Can you work these out from the model? Positions are in its coordinate system, mm. Face numbers are marked on the shaded views. A direction names the side the tool comes from. Give positions to 0.01 mm unless a question says otherwise; leave off trailing zeros. Loops run counter-clockwise (first coordinate to the right, second up) from the corner with the lowest first, then second, coordinate; pieces in that order, holes last. Notation, with made-up numbers: (36.25, 38.25) - (68.25, 38.25) arc R13 cw to (68.25, 63.25) - close; hole circle Ø7 at (71.5, 38.5). An arc over 180 degrees is marked (long way). Answer as a JSON object with one key per item and string values. Group by question number.
Item 1: Suppose I cut it at C-C on y = 0.5. Count the separate pieces of the cut face and the enclosed holes in it, and give its area (3 significant figures).
Item 2: Suppose I cut it at D-D on z = 8.5. Write out the boundary of the cut face in (x, y), and give its area (3 significant figures).
Item 3: Thinking about a two-plate mould opening in X: for the marked faces 4, 5 and 6, which applies, pulls with the +X half, pulls with the -X half, needs draft (parallel to the pull), parting line crosses it, or undercut?
Item 4: Will these pins go through, and if not, where does the flat tip stop? pin 1 (10 mm diameter, centred on x = 12, z = 17.5, fed in from -Y); pin 2 (1.5 mm diameter, centred on x = 0, y = -15, fed in from -Z); pin 3 (8 mm diameter, centred on y = 6.5, z = 17.5, fed in from +X); pin 4 (4 mm diameter, centred on x = 1, z = 16.5, fed in from -Y).
Item 5: Suppose I cut it at B-B on z = 10.75. Write out the boundary of the cut face in (x, y), and give its area (3 significant figures).
Item 6: Please list where these lines run through material, in increasing order: L1, parallel to Y at x = 0, z = 1.95; L2, parallel to Z at x = 4.5, y = 5.5; L3, parallel to Y at x = -0.5, z = 19.25.
Item 7: Which directions (+Z, -Z, +X, -X, +Y, -Y) give clear straight access to the entire face, cutting with the end or side of a thin tool? Please do the marked faces 1, 2 and 3.
Item 8: Suppose I cut it at A-A on x = 0. Write out the boundary of the cut face in (y, z), and give its area (3 significant figures).
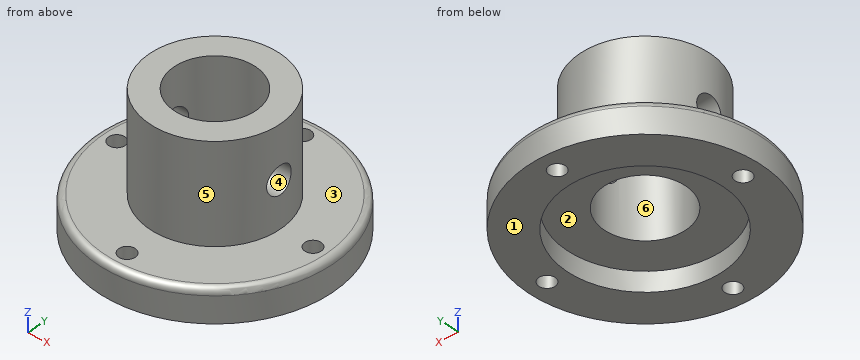
from build123d import *

# Parameters (mm, degrees)
SKETCH_1_R               = 18
SKETCH_1_R_2             = 12
SKETCH_1_R_3             = 1.25
EXTRUDE_1_DEPTH          = 5
EXTRUDE_START            = -2
SKETCH_2_R               = 12
SKETCH_2_R_2             = 10
EXTRUDE_2_DEPTH          = 2
FILLET_1_R               = 1
SKETCH_3_R               = 10
SKETCH_3_R_2             = 6.25
EXTRUDE_3_DEPTH          = 17
CUT_EXTRUDE_1_DEPTH      = 20
CUT_EXTRUDE_1_DEPTH_BACK = 20
SKETCH_4_R               = 2.1


with BuildPart() as part:
    # Sketch 1 → Extrude 1 (new body)
    with BuildSketch(Plane.XY):
        Circle(SKETCH_1_R)
        Circle(SKETCH_1_R_2, mode=Mode.SUBTRACT)
        with Locations((0, 15)):
            Circle(SKETCH_1_R_3, mode=Mode.SUBTRACT)
        with Locations((-15, 0)):
            Circle(SKETCH_1_R_3, mode=Mode.SUBTRACT)
        with Locations((0, -15)):
            Circle(SKETCH_1_R_3, mode=Mode.SUBTRACT)
        with Locations((15, 0)):
            Circle(SKETCH_1_R_3, mode=Mode.SUBTRACT)
    extrude(amount=EXTRUDE_1_DEPTH)

    # Sketch 2 → Extrude 2 (add)
    with BuildSketch(Plane.XY.offset(5).offset(EXTRUDE_START)):
        Circle(SKETCH_2_R)
        Circle(SKETCH_2_R_2, mode=Mode.SUBTRACT)
    extrude(amount=EXTRUDE_2_DEPTH)

    # Fillet 1
    fillet_1_edges = [part.edges().sort_by_distance(p)[0] for p in [
        (-18, 0, 5),
    ]]
    fillet(fillet_1_edges, radius=FILLET_1_R)

    # Sketch 3 → Extrude 3 (add)
    with BuildSketch(Plane(origin=(0, 0, 3), x_dir=(-1, 0, 0), z_dir=(0, 0, -1))):
        Circle(SKETCH_3_R)
        Circle(SKETCH_3_R_2, mode=Mode.SUBTRACT)
    extrude(amount=-EXTRUDE_3_DEPTH)

    # Sketch 4 → Cut-Extrude 1 (cut, two sides: drawn at the far end of the back side and taken through both)
    with BuildSketch(Plane(origin=(0, 0, 0), x_dir=(0, 0, -1), z_dir=(1, 0, 0)).offset(-CUT_EXTRUDE_1_DEPTH_BACK)):
        with Locations(Location((-12, 0, 0), (0, 0, 180))):
            Circle(SKETCH_4_R)
    extrude(amount=CUT_EXTRUDE_1_DEPTH + CUT_EXTRUDE_1_DEPTH_BACK, mode=Mode.SUBTRACT)


solid = part.part
Worked out:
{
 "1": {"separate pieces": "6", "enclosed holes": "0", "area": "142 mm2"},
 "2": {"outline": "circle Ø20 at (0, 0); hole circle Ø12.5 at (0, 0)", "area": "191 mm2"},
 "3": {"face 4": "needs draft", "face 5": "parting line crosses it", "face 6": "undercut"},
 "4": {"pin 1": "stops at y = -7.14", "pin 2": "passes through", "pin 3": "stops at x = 9.68", "pin 4": "stops at y = -10"},
 "5": {"outline": "(-9.86, -1.69) arc R10 ccw to (9.86, -1.69) - (6.02, -1.69) arc R6.25 cw to (-6.02, -1.69) - close; (-9.86, 1.69) - (-6.02, 1.69) arc R6.25 cw to (6.02, 1.69) - (9.86, 1.69) arc R10 ccw to start", "area": "166 mm2"},
 "6": {"L1": "y = -18 to -16.25, -13.75 to -12, 12 to 13.75, 16.25 to 18", "L2": "z = 3 to 20", "L3": "y = -9.99 to -6.23, 6.23 to 9.99"},
 "7": {"face 1": "-Z, +X, -X, +Y, -Y", "face 2": "-Z", "face 3": "+Z"},
 "8": {"outline": "(-18, 0) - (-16.25, 0) - (-16.25, 5) - (-17, 5) arc R1 ccw to (-18, 4) - close; (-13.75, 0) - (-12, 0) - (-12, 3) - (-6.25, 3) - (-6.25, 20) - (-10, 20) - (-10, 5) - (-13.75, 5) - close; (6.25, 3) - (12, 3) - (12, 0) - (13.75, 0) - (13.75, 5) - (10, 5) - (10, 20) - (6.25, 20) - close; (16.25, 0) - (18, 0) - (18, 4) arc R1 ccw to (17, 5) - (16.25, 5) - close", "area": "170 mm2"}
}
